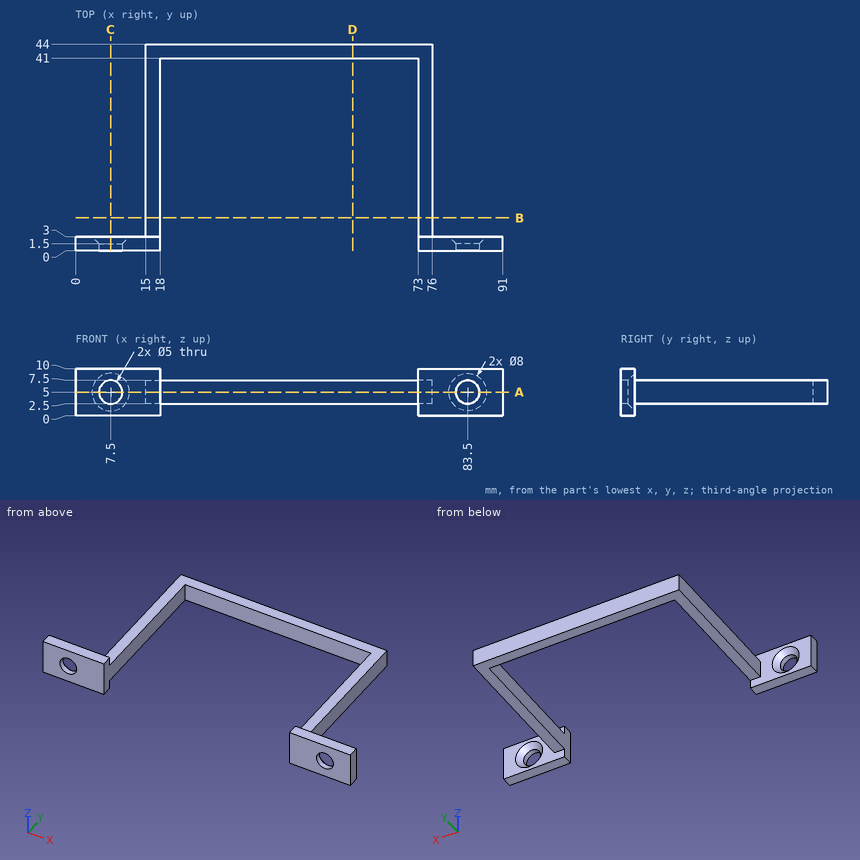
Part print with two shaded views. Sizes in mm from the minimum x, y, z corner. Give positions to 0.01 mm unless a question says otherwise; leave off trailing zeros. Order: outer loops, then holes, each group sorted by start corner. A loop starts at its lowest first (then second) coordinate and runs counter-clockwise, first axis right, second up.
1) Wall check: probe 1 along X at (y, z) = (1, 5); probe 2 along X at (y, z) = (36, 5); probe 3 along Z at (x, y) = (83.5, 0.85). Give the ranges that are in metal, low to high.
2) Saw through at B-B, the plane y = 7. Write the cut outline in (x, z).
3) Saw through at C-C, the plane x = 7.5. Write the cut outline in (y, z), then the cut area to 4 significant figures.
4) Pin check, flat tips, straight feed: pin 1 (1.5 mm diameter, centred on y = 24, z = 5.5, fed in from +X); pin 2 (1 mm diameter, centred on y = 35.5, z = 6.5, fed in from -X); pin 3 (5.5 mm diameter, centred on x = 57, z = 5, fed in from -Y). Stop position of each tip, or through.
5) Saw through at A-A, the plane z = 5. Write the cut outline in (x, y), then the cut area to 4 significant figures.
6) Saw through at D-D, the plane x = 59. Write the cut outline in (y, z), then the cut area to 3 significant figures.
Computed:
1. probe 1: x = 0 to 5, 10 to 18, 73 to 81, 86 to 91
1. probe 2: x = 15 to 18, 73 to 76
1. probe 3: z = 0 to 2.5, 7.5 to 10
2. outline: (15, 2.5) - (18, 2.5) - (18, 7.5) - (15, 7.5) - close; (73, 2.5) - (76, 2.5) - (76, 7.5) - (73, 7.5) - close
3. outline: (0, 0) - (3, 0) - (3, 1) - (1.5, 2.5) - (0, 2.5) - close; (0, 7.5) - (1.5, 7.5) - (3, 9) - (3, 10) - (0, 10) - close
3. area: 12.75 mm2
4. pin 1: stops at x = 76
4. pin 2: stops at x = 15
4. pin 3: stops at y = 41
5. outline: (0, 0) - (5, 0) - (5, 1.5) - (3.5, 3) - (0, 3) - close; (10, 0) - (18, 0) - (18, 41) - (73, 41) - (73, 0) - (81, 0) - (81, 1.5) - (79.5, 3) - (76, 3) - (76, 44) - (15, 44) - (15, 3) - (11.5, 3) - (10, 1.5) - close; (86, 0) - (91, 0) - (91, 3) - (87.5, 3) - (86, 1.5) - close
5. area: 484.5 mm2
6. outline: (41, 2.5) - (44, 2.5) - (44, 7.5) - (41, 7.5) - close
6. area: 15.0 mm2
